Here's how the part is built. I have some questions about the finished solid (model axes, mm). Face numbers are marked on the shaded views. Round coordinates to 2 decimals unless told otherwise and drop trailing zeros. Loops run counter-clockwise (first coordinate to the right, second up) from the corner with the lowest first, then second, coordinate; pieces in that order, holes last. Notation, with made-up numbers: M -39.75,14 L 14.25,14 A33 cw 14.25,42 Z; hole C 11,81 d11. An arc over 180 degrees is marked long. Answer as a JSON object with one key per item and string values.
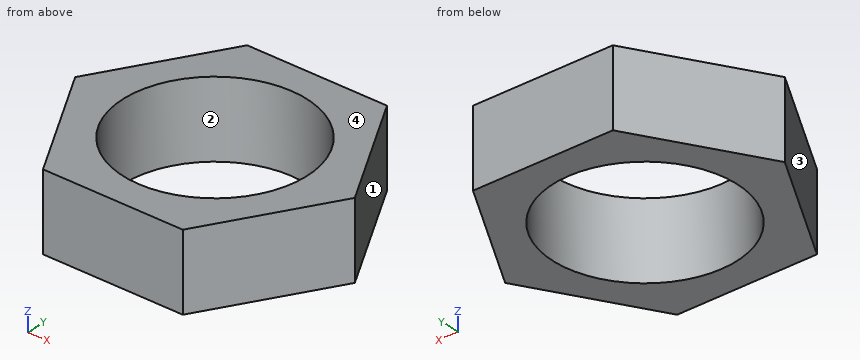
Autodesk Inventor part; units mm, degrees
ref_plane "YZ Plane" through (0, 0, 0) normal (1, 0, 0) x (0, 1, 0)
ref_plane "XZ Plane" through (0, 0, 0) normal (0, 1, 0) x (-1, 0, 0)
ref_plane "XY Plane" through (0, 0, 0) normal (0, 0, 1) x (1, 0, 0)
sketch "Sketch1" plane through (0, 0, 0) normal (0, 0, 1) x (1, 0, 0)
  line L0 (234.6351, 0) -> (117.3176, -203.2)
  line L1 (117.3176, -203.2) -> (-117.3176, -203.2)
  line L2 (-117.3176, -203.2) -> (-234.6351, 0)
  line L3 (-234.6351, 0) -> (-117.3176, 203.2)
  line L4 (-117.3176, 203.2) -> (117.3176, 203.2)
  line L5 (117.3176, 203.2) -> (234.6351, 0)
  circle A0 centre (0, 0) radius 152.4
  point P0 (0, -203.2)
  point P1 (0, 203.2)
  dimension "d0" = 406.4
  dimension "d1" = 304.8
extrude "Extrusion1" add sketch "Sketch1" along normal blind 127
properties part number "Bolt"
Item 1: I want a section at C-C on y = 144. List the corners of the cut face in (x, z) for me, plus the area to 3 significant figures.
Solution:
{"outline": "M -151.5,0 L -49.9,0 L -49.9,127 L -151.5,127 Z; M 49.9,0 L 151.5,0 L 151.5,127 L 49.9,127 Z", "area": "25,800 mm2"}
Item 2: For P1, Ø12, axis at y = -40.5, z = 37, coming from the +X side; P2, Ø1.5, axis at y = -111, z = 43, coming from the -X side; P3, Ø2, axis at y = -19, z = 85.5, coming from the +X side, each with a flat end and sliding along its axis, tell me the tip position at first contact or that it passes through.
Solution:
{"P1": "stops at x = 214.72", "P2": "stops at x = -170.98", "P3": "stops at x = 224.24"}
Item 3: We'd pull the mould along Y, two halves only. Please class the marked faces 1, 2, 3 and 4: +Y half, -Y half, draft (parallel to the pull), parting line (faces both ways), or undercut.
Solution:
{"face 1": "+Y half", "face 2": "undercut", "face 3": "-Y half", "face 4": "draft"}
Item 4: If I drill on L1, parallel to Y at x = 0, z = 77; L2, parallel to X at y = -41, z = 6; L3, parallel to Y at x = 79, z = 101.5, over which ranges is the centre line in solid material (lowest first)? Write a range as from..to.
Solution:
{"L1": "y = -203.2..-152.4, 152.4..203.2", "L2": "x = -210.96..-146.78, 146.78..210.96", "L3": "y = -203.2..-130.33, 130.33..203.2"}
Item 5: I want a section at B-B on z = 14.5. List the corners of the cut face in (x, y) for me.
Solution:
{"outline": "M -234.64,0 L -117.32,-203.2 L 117.32,-203.2 L 234.64,0 L 117.32,203.2 L -117.32,203.2 Z; hole C 0,0 d304.8"}
Item 6: I want a section at A-A on x = 0. List the corners of the cut face in (y, z) for me, plus the area to 3 significant figures.
Solution:
{"outline": "M -203.2,0 L -152.4,0 L -152.4,127 L -203.2,127 Z; M 152.4,0 L 203.2,0 L 203.2,127 L 152.4,127 Z", "area": "12,900 mm2"}
